Design review of the part built by this model. Coordinates are the model's own, in mm. A direction names the side the tool comes from. Round coordinates to 2 decimals unless told otherwise and drop trailing zeros. Loops run counter-clockwise (first coordinate to the right, second up) from the corner with the lowest first, then second, coordinate; pieces in that order, holes last. Notation, with made-up numbers: (-2.5, 72.5) -> (41.5, 72.5) arc R12 cw to (41.5, 81.5) -> close; hole circle Ø2 at (-27, 87). An arc over 180 degrees is marked (long way). Write each question's results on one line, items separated by ' | '. Start each with the question number.
Autodesk Inventor part; units mm, degrees
ref_plane "YZ Plane" through (0, 0, 0) normal (1, 0, 0) x (0, 1, 0)
ref_plane "XZ Plane" through (0, 0, 0) normal (0, 1, 0) x (-1, 0, 0)
ref_plane "XY Plane" through (0, 0, 0) normal (0, 0, 1) x (1, 0, 0)
sketch "Sketch1" plane through (0, 0, 0) normal (0, 0, 1) x (1, 0, 0)
  line L0 (-12.7, 528.7976) -> (-12.7, -380.5224)
  line L1 (12.7, 528.7976) -> (12.7, -380.5224)
  circle A0 centre (-30.0251, 19.05) radius 2.3813
  circle A1 centre (-30.0251, 0) radius 2.3813
  circle A2 centre (-30.0251, -19.05) radius 2.3813
  line L2 (-14.1501, -31.886) -> (-58.6001, -31.886)
  line L3 (-58.6001, -31.886) -> (-58.6001, 33.5086)
  line L4 (-58.6001, 33.5086) -> (-14.1501, 33.5086)
  line L5 (-14.1501, 33.5086) -> (-14.1501, -31.886)
  line L6 (-25.1651, -297.4161) -> (-25.1651, -366.8339)
  point P0 (0, 0)
  dimension "d0" = 15.875
  dimension "d1" = 28.575
extrude "Extrusion1" add sketch "Sketch1" along normal blind 33.655
sketch "Sketch2" plane through (0, 0, 33.655) normal (0, 0, 1) x (1, 0, 0)
  circle A0 centre (-30.0251, -19.05) radius 2.3813
  circle A1 centre (-30.0251, 0) radius 2.3813
  circle A2 centre (-30.0251, 19.05) radius 2.3813
  point P0 (0, 0)
extrude "Extrusion2" add sketch "Sketch2" against normal blind 6.35
sketch "Sketch3" plane through (0, 0, 33.655) normal (0, 0, 1) x (1, 0, 0)
  circle A0 centre (-52.2501, -25.536) radius 2.3813
  line L0 (-58.6001, 33.5086) -> (-58.6001, -31.886) construction
  line L1 (-58.6001, 0) -> (-1.0342, 0) construction
  line L2 (-58.6001, -31.886) -> (-14.1501, -31.886) construction
  line L3 (-36.3751, -31.886) -> (-36.3751, 36.9987) construction
  circle A1 centre (-30.0251, -19.05) radius 2.3813 construction
  circle A2 centre (-30.0251, 0) radius 2.3813 construction
  circle A3 centre (-30.0251, 19.05) radius 2.3813 construction
  circle A4 centre (-52.2501, 25.536) radius 2.3813
  circle A5 centre (-20.5001, -25.536) radius 2.3813
  circle A6 centre (-20.5001, 25.536) radius 2.3813
  point P0 (0, 0)
  dimension "d6" = 4.7625
  dimension "d7" = 6.35
  dimension "d8" = 6.35
extrude "Extrusion3" cut sketch "Sketch3" against normal blind 19.05
sketch "Sketch4" plane through (0, 0, 33.655) normal (0, 0, 1) x (1, 0, 0)
  point P0 (0, 0)
properties part number "Transmission Clamp"
1) The part is to be moulded in two halves that separate along Y. For faces 1 (the face through (-37, 33.509, 17)), 2 (the face through (-58.6, 0, 17)), 3 (the face through (-21, 26, 14.605)), say which applies: +Y half, -Y half, draft (parallel to the pull), parting line (faces both ways), or undercut.
2) Take a section at A-A (z = 6). Write out the cut boundary in (x, y), plus the area to 3 significant figures.
3) Take a section at B-B (y = -19.05). Write out the cut boundary in (x, z) (3 decimals).
4) Take a section at C-C (x = -53.5). Write out the cut boundary in (y, z) (3 decimals).
5) Insertion check: pin 1 (4 mm diameter, centred on x = -29.5, y = -19.5, fed in from -Z); pin 2 (3 mm diameter, centred on x = -30.03, y = 0, fed in from -Z) (3 decimals); pin 3 (1.4 mm diameter, centred on x = -51.5, y = -25.5, fed in from +Z) (3 decimals). Each pin has a flat end and moves straight along its axis. Give the tip position at first contact, or say it passes through.
6) To check wall thickness, follow line 1 (X direction, y = -19, z = 10); line 2 (Z direction, x = -32, y = 0) (3 decimals); line 3 (X direction, y = 1, z = 10.5). State the ranges of each line that lie inside material, in increasing order. Write a range as from..to.
7) Take a section at D-D (y = 17.5). Write out the cut boundary in (x, z) (3 decimals), plus the area to 3 significant figures.
8) For faces 4 (the face through (-21.016, 23.211, 24.263)), 5 (the face through (-37, 1, 0)), 6 (the face through (-32.4, -19.2, 13.5)), list the 3-axis set-ups (+Z, -Z, +X, -X, +Y, -Y) from which the entire face can be reached by the end or side of a thin tool; tool diameter is ignored.
Geometry check:
1) face 1: +Y half | face 2: draft | face 3: undercut
2) outline: (-58.6, -31.89) -> (-14.15, -31.89) -> (-14.15, 33.51) -> (-58.6, 33.51) -> close; hole circle Ø4.76 at (-30.03, -19.05); hole circle Ø4.76 at (-30.03, 0); hole circle Ø4.76 at (-30.03, 19.05) | area: 2,850 mm^2
3) outline: (-58.6, 0) -> (-32.406, 0) -> (-32.406, 27.305) -> (-27.644, 27.305) -> (-27.644, 0) -> (-14.15, 0) -> (-14.15, 33.655) -> (-58.6, 33.655) -> close
4) outline: (-31.886, 0) -> (33.509, 0) -> (33.509, 33.655) -> (27.563, 33.655) -> (27.563, 14.605) -> (23.509, 14.605) -> (23.509, 33.655) -> (-23.509, 33.655) -> (-23.509, 14.605) -> (-27.563, 14.605) -> (-27.563, 33.655) -> (-31.886, 33.655) -> close
5) pin 1: stops at z = 0 | pin 2: stops at z = 27.305 | pin 3: stops at z = 14.605
6) line 1: x = -58.6..-32.41, -27.64..-14.15 | line 2: z = 27.305..33.655 | line 3: x = -58.6..-32.19, -27.86..-14.15
7) outline: (-58.6, 0) -> (-31.833, 0) -> (-31.833, 27.305) -> (-28.217, 27.305) -> (-28.217, 0) -> (-14.15, 0) -> (-14.15, 33.655) -> (-58.6, 33.655) -> close | area: 1,400 mm^2
8) face 4: +Z | face 5: -Z, +X, -X, +Y, -Y | face 6: -Z
